Geometry check sheet. Reference: the model listing, model coordinates, mm. A direction names the side the tool comes from. Round coordinates to 2 decimals unless told otherwise and drop trailing zeros. Order: outer loops, then holes, each group sorted by start corner. A loop starts at its lowest first (then second) coordinate and runs counter-clockwise, first axis right, second up.
```python
from build123d import *

# Parameters (mm, degrees)
SKETCH_1_W      = 22.7
SKETCH_1_H      = 10.1
EXTRUDE_1_DEPTH = 10
SKETCH_2_W      = 3.6
SKETCH_2_H      = 4.6
SKETCH_2_R      = 1.15
EXTRUDE_2_DEPTH = 3.8


with BuildPart() as part:
    # ｽｹｯﾁ1 → ﾎﾞｽ - 押し出し1 (new body)
    with BuildSketch(Plane(origin=(0, 0, 0), x_dir=(1, 0, 0), z_dir=(0, 1, 0))):
        with Locations((11.35, 5.05)):
            Rectangle(SKETCH_1_W, SKETCH_1_H)
    extrude(amount=EXTRUDE_1_DEPTH)

    # ｽｹｯﾁ2 → ﾎﾞｽ - 押し出し2 (add)
    # profile 1 of 2: a face of its own
    with BuildSketch(Plane.XZ):
        with Locations((-1.8, -5.05)):
            Rectangle(SKETCH_2_W, SKETCH_2_H)
        with Locations(Location((-1.8, -5.05, 0), (0, 0, 270))):
            Circle(SKETCH_2_R, mode=Mode.SUBTRACT)
    # profile 2 of 2: a face of its own
    with BuildSketch(Plane.XZ):
        with Locations((24.5, -5.05)):
            Rectangle(SKETCH_2_W, SKETCH_2_H)
        with Locations(Location((24.5, -5.05, 0), (0, 0, 270))):
            Circle(SKETCH_2_R, mode=Mode.SUBTRACT)
    extrude(amount=-EXTRUDE_2_DEPTH)


solid = part.part
```
(1) Sectioned sample at D-D, the plane z = -6.75. Record the cut outline in (x, y), and give its area (3 significant figures).
Returned:
outline: (-3.6, 0) - (26.3, 0) - (26.3, 3.8) - (22.7, 3.8) - (22.7, 10) - (0, 10) - (0, 3.8) - (-3.6, 3.8) - close
area: 254 mm2
(2) Set-up check for faces 1 (the flat face through (24, 2, -7.35)), 2 (the flat face through (26, 3.8, -5)), 3 (the flat face through (24, 2, -2.75)), 4 (the flat face through (-3, 3.8, -4)): record each of +Z, -Z, +X, -X, +Y, -Y from which the full face is reachable in a straight line by a thin tool's end or side.
Returned:
face 1: -Z, +X, +Y, -Y
face 2: +Z, -Z, +X, +Y
face 3: +Z, +X, +Y, -Y
face 4: +Z, -Z, -X, +Y
(3) Sectioned sample at B-B, the plane z = -5.05. Record the cut outline in (x, y), and give its area (3 significant figures).
Returned:
outline: (-3.6, 0) - (-2.95, 0) - (-2.95, 3.8) - (-3.6, 3.8) - close; (-0.65, 0) - (23.35, 0) - (23.35, 3.8) - (22.7, 3.8) - (22.7, 10) - (0, 10) - (0, 3.8) - (-0.65, 3.8) - close; (25.65, 0) - (26.3, 0) - (26.3, 3.8) - (25.65, 3.8) - close
area: 237 mm2
(4) Material ranges on line 1 (X direction, y = 1.2, z = -5.05); line 2 (X direction, y = 1.25, z = -4); line 3 (X direction, y = 1.25, z = -7.75), recorded low to high.
Returned:
line 1: x = -3.6 to -2.95, -0.65 to 23.35, 25.65 to 26.3
line 2: x = -3.6 to -2.27, -1.33 to 24.03, 24.97 to 26.3
line 3: x = 0 to 22.7
(5) Sectioned sample at A-A, the plane x = -1.8. Record the cut outline in (y, z).
Returned:
outline: (0, -7.35) - (3.8, -7.35) - (3.8, -6.2) - (0, -6.2) - close; (0, -3.9) - (3.8, -3.9) - (3.8, -2.75) - (0, -2.75) - close
(6) Sectioned sample at C-C, the plane y = 2.5. Record the cut outline in (x, z).
Returned:
outline: (-3.6, -7.35) - (0, -7.35) - (0, -10.1) - (22.7, -10.1) - (22.7, -7.35) - (26.3, -7.35) - (26.3, -2.75) - (22.7, -2.75) - (22.7, 0) - (0, 0) - (0, -2.75) - (-3.6, -2.75) - close; hole circle Ø2.3 at (-1.8, -5.05); hole circle Ø2.3 at (24.5, -5.05)
(7) Depth check by flat-ended pin: P1, Ø1.1, axis at x = 25.5, y = 2.5, coming from the +Z side; P2, Ø1.8, axis at x = -2, z = -5, coming from the +Y side; P3, Ø1.1, axis at x = 25, y = 2, coming from the -Z side; P4, Ø3, axis at x = -1.8, z = -5.05, coming from the +Y side. Enter the tip coordinate at first touch or a pass-through.
Returned:
P1: stops at z = -2.75
P2: passes through
P3: stops at z = -7.35
P4: stops at y = 3.8
(8) Draft check along Z on faces 5 (the cylindrical face through (-1.455, 1.873, -6.147)), 6 (the flat face through (11, 0, -5)), 7 (the flat face through (-2, 2, -2.75)). Enter one of: released by +Z, released by -Z, zero draft, split by the parting line, or undercut.
Returned:
face 5: undercut
face 6: zero draft
face 7: released by +Z
